Part model, mm, in its own coordinate system. A direction names the side the tool comes from. Round coordinates to 2 decimals unless told otherwise and drop trailing zeros. Write each loop counter-clockwise with the first axis right and the second up, starting at its lowest first coordinate (ties: lowest second). Pieces come first, ordered by that corner, then holes. Notation, with made-up numbers: M 80.5,85.5 L 125.5,85.5 A20 cw 125.5,91.5 Z; hole C 5,-27 d4. An arc over 180 degrees is marked long. Use a Markdown table: item, result. Add a question column.
1) Drop flat-ended pins along their axis: P1, Ø12, axis at x = 69.5, y = 14.5, coming from the -Z side; P2, Ø6, axis at x = 12.7, y = 25.4, coming from the +Z side. Give the stop position or say it passes through.
2) Wall check: probe 1 along Y at (x, z) = (76.2, 2.25); probe 2 along X at (y, z) = (15.5, -18) (3 decimals); probe 3 along X at (y, z) = (6, 1). Give the ranges that are in metal, low to high.
3) Slice it at B-B on z = -36. Write the cut outline in (x, y) (3 decimals).
4) Slice it at D-D on y = 11. Write the cut outline in (x, z) (3 decimals), plus the area to 3 significant figures.
5) Two-plate mould, pull along Y, no slides. Class faces 1 (the face through (-3, 16, -47.625)), 2 (the face through (44.2, 0, 0.2)), 3 (the face through (73.58, 27.41, 1.57)): released by +Y, released by -Y, zero draft, split by the parting line, or undercut.
6) Which spindle directions (+Z, -Z, +X, -X, +Y, -Y) get a long thin tool onto all of the face, cutting with end or side? Do faces 4 (the face through (-1.27, 16, -24)), 5 (the face through (44.7, 31.75, 0.2)). Say none if no direction does.
7) Slice it at A-A on y = 6.35. Write the cut outline in (x, z) (3 decimals), plus the area to 3 significant figures.
8) Slice it at C-C on x = 13.5. Write the cut outline in (y, z) (3 decimals).
Autodesk Inventor part; units mm, degrees
ref_plane "YZ Plane" through (0, 0, 0) normal (1, 0, 0) x (0, 1, 0)
ref_plane "XZ Plane" through (0, 0, 0) normal (0, 1, 0) x (-1, 0, 0)
ref_plane "XY Plane" through (0, 0, 0) normal (0, 0, 1) x (1, 0, 0)
sketch "Sketch1" plane through (0, 0, 0) normal (0, 0, 1) x (1, 0, 0)
  line L0 (0, 0) -> (88.9, 0)
  line L1 (88.9, 0) -> (88.9, 31.75)
  line L2 (88.9, 31.75) -> (0, 31.75)
  line L3 (0, 31.75) -> (0, 0)
  circle A0 centre (12.7, 25.4) radius 3.302
  circle A1 centre (76.2, 25.4) radius 3.302
  circle A2 centre (12.7, 6.35) radius 3.302
  circle A3 centre (76.2, 6.35) radius 3.302
  line L4 (12.7, 25.4) -> (76.2, 25.4) construction
  line L5 (44.45, 31.75) -> (44.45, 0) construction
  point P0 (44.45, 25.4)
  dimension "d0" = 88.9
  dimension "d2" = 31.75
  dimension "d5" = 63.5
  dimension "d8" = 19.05
  dimension "d11" = 6.35
  dimension "d12" = 6.604
extrude "Plate1" add sketch "Sketch1" along normal blind 3.175
sketch "Sketch2" plane through (90.17, 0, -1.27) normal (1, 0, 0) x (0, 1, 0)
  line L0 (31.75, 0) -> (0, 0)
  line L1 (0, 0) -> (0, -46.355)
  line L2 (0, -46.355) -> (31.75, -46.355)
  line L3 (31.75, -46.355) -> (31.75, 0)
edge flange "Flange1" height 50.8 angle 90 thickness 3.175 bend radius 1.27 thickness toward (1, 0, 0) relief straight relief width 3.175 relief depth 1.5875 corner gap 3.175 corner form 0 edges at (88.9, 15.875, 0) (0, 15.875, 0) wall of the first edge with corners at (90.17, 31.75, -1.27) (90.17, 0, -1.27) (90.17, 0, -47.625) (90.17, 31.75, -47.625)
bend "Bend1"
corner "Corner1"
equation "\"d16\" = BendReliefWidth"
equation "\"d17\" = BendReliefDepth"
equation "\"d18\" = MinimumRemnant"
equation "\"d19\" = BendRadius"
equation "\"d23\" = CornerReliefSize"
equation "\"d24\" = GapSize"
equation "\"d25\" = JacobiRadiusSize"
equation "\"BendRadius\" = Thickness"
equation "\"BendReliefWidth\" = Thickness"
equation "\"BendReliefDepth\" = 0.5 * Thickness"
equation "\"CornerReliefSize\" = 4 * Thickness"
equation "\"MinimumRemnant\" = 2 * Thickness"
equation "\"TransitionRadius\" = BendRadius"
equation "\"JacobiRadiusSize\" = Thickness"
equation "\"GapSize\" = Thickness"
equation "\"d15\" = BendRadius"
properties part number "M - Upper Rail Connector Bracket 1" material "Aluminum 6061"
Entries:
| question | item | result |
|---|---|---|
| 1 | P1 | stops at z = 0 |
| 1 | P2 | passes through |
| 2 | probe 1 | y = 0 to 3.05, 9.65 to 22.1, 28.7 to 31.75 |
| 2 | probe 2 | x = -4.445 to -1.27, 90.17 to 93.345 |
| 2 | probe 3 | x = -3.82 to 9.42, 15.98 to 72.92, 79.48 to 92.72 |
| 3 | outline | M -4.445,0 L -1.27,0 L -1.27,31.75 L -4.445,31.75 Z; M 90.17,0 L 93.345,0 L 93.345,31.75 L 90.17,31.75 Z |
| 4 | outline | M -4.445,-47.625 L -1.27,-47.625 L -1.27,-1.27 A1.27 cw 0,0 L 88.9,0 A1.27 cw 90.17,-1.27 L 90.17,-47.625 L 93.345,-47.625 L 93.345,-1.27 A4.445 ccw 88.9,3.175 L 0,3.175 A4.445 ccw -4.445,-1.27 Z |
| 4 | area | 605 mm^2 |
| 5 | face 1 | zero draft |
| 5 | face 2 | released by -Y |
| 5 | face 3 | undercut |
| 6 | face 4 | -Z, +Y, -Y |
| 6 | face 5 | +Z, -Z, +X, -X, +Y |
| 7 | outline | M -4.445,-47.625 L -1.27,-47.625 L -1.27,-1.27 A1.27 cw 0,0 L 9.398,0 L 9.398,3.175 L 0,3.175 A4.445 ccw -4.445,-1.27 Z; M 16.002,0 L 72.898,0 L 72.898,3.175 L 16.002,3.175 Z; M 79.502,0 L 88.9,0 A1.27 cw 90.17,-1.27 L 90.17,-47.625 L 93.345,-47.625 L 93.345,-1.27 A4.445 ccw 88.9,3.175 L 79.502,3.175 Z |
| 7 | area | 563 mm^2 |
| 8 | outline | M 0,0 L 3.146,0 L 3.146,3.175 L 0,3.175 Z; M 9.554,0 L 22.196,0 L 22.196,3.175 L 9.554,3.175 Z; M 28.604,0 L 31.75,0 L 31.75,3.175 L 28.604,3.175 Z |
